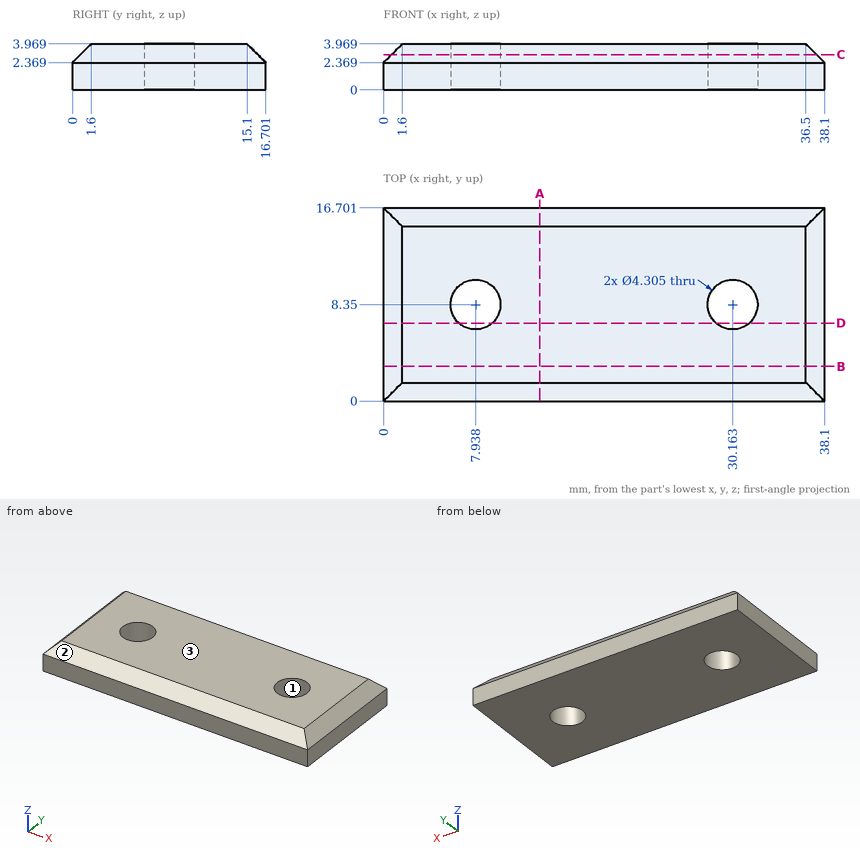
Check sheet for the drawn part. Datum: minimum x, y, z corner. Units: mm. Round coordinates to 2 decimals unless told otherwise and drop trailing zeros. Loops run counter-clockwise (first coordinate to the right, second up) from the corner with the lowest first, then second, coordinate; pieces in that order, holes last.
Item 1: Cross-section at D-D on y = 6.75. Record the boundary of the cut face in (x, z), then the cut area to 3 significant figures.
Item 2: Cross-section at A-A on x = 13.5. Record the boundary of the cut face in (y, z).
Item 3: Thickness scan on line 1 (Y direction, x = 8, z = 1.2); line 2 (X direction, y = 7, z = 3) (1 decimal); line 3 (Y direction, x = 6, z = 0.6) (1 decimal). Record the ranges inside material, lowest first.
Item 4: Mould release check, pull along Y, two halves, no side actions. Record for the marked faces 1, 2 and 3: pulls with the +Y half, pulls with the -Y half, needs draft (parallel to the pull), parting line crosses it, or undercut.
Item 5: Cross-section at B-B on y = 3. Record the boundary of the cut face in (x, z), then the cut area to 3 significant figures.
Item 6: Cross-section at C-C on z = 3.05. Count the separate pieces of the cut face and the enclosed holes in it, then the cut area to 3 significant figures.
Answer sheet:
1. outline: (0, 0) - (6.5, 0) - (6.5, 3.97) - (1.6, 3.97) - (0, 2.37) - close; (9.38, 0) - (28.72, 0) - (28.72, 3.97) - (9.38, 3.97) - close; (31.6, 0) - (38.1, 0) - (38.1, 2.37) - (36.5, 3.97) - (31.6, 3.97) - close
1. area: 126 mm2
2. outline: (0, 0) - (16.7, 0) - (16.7, 2.37) - (15.1, 3.97) - (1.6, 3.97) - (0, 2.37) - close
3. line 1: y = 0 to 6.2, 10.5 to 16.7
3. line 2: x = 0.6 to 6.3, 9.6 to 28.5, 31.8 to 37.5
3. line 3: y = 0 to 7.4, 9.3 to 16.7
4. face 1: undercut
4. face 2: pulls with the -Y half
4. face 3: needs draft
5. outline: (0, 0) - (38.1, 0) - (38.1, 2.37) - (36.5, 3.97) - (1.6, 3.97) - (0, 2.37) - close
5. area: 149 mm2
6. separate pieces: 1
6. enclosed holes: 2
6. area: 534 mm2
